Autodesk Inventor part; units mm, degrees
ref_plane "YZ Plane" through (0, 0, 0) normal (1, 0, 0) x (0, 1, 0)
ref_plane "XZ Plane" through (0, 0, 0) normal (0, 1, 0) x (-1, 0, 0)
ref_plane "XY Plane" through (0, 0, 0) normal (0, 0, 1) x (1, 0, 0)
sketch "Sketch1" plane through (0, 0, 0) normal (0, 0, 1) x (1, 0, 0)
  circle A0 centre (15.5, -15.5) radius 2
  circle A1 centre (-15.5, -15.5) radius 2
  circle A2 centre (15.5, 15.5) radius 2
  circle A3 centre (-15.5, 15.5) radius 2
  line L0 (-21.15, 15.4985) -> (-15.4985, 21.15)
  line L1 (-15.4985, 21.15) -> (15.4985, 21.15)
  line L2 (15.4985, 21.15) -> (21.15, 15.4985)
  line L3 (21.15, 15.4985) -> (21.15, -15.4985)
  line L4 (21.15, -15.4985) -> (15.4985, -21.15)
  line L5 (15.4985, -21.15) -> (-15.4985, -21.15)
  line L6 (-15.4985, -21.15) -> (-21.15, -15.4985)
  line L7 (-21.15, -15.4985) -> (-21.15, 15.4985)
  line L8 (28.575, -18.574) -> (28.575, 18.574)
  line L9 (28.575, 18.574) -> (18.574, 28.575)
  line L10 (18.574, 28.575) -> (-18.574, 28.575)
  line L11 (-18.574, 28.575) -> (-28.575, 18.574)
  line L12 (-28.575, 18.574) -> (-28.575, -18.574)
  line L13 (-28.575, -18.574) -> (-18.574, -28.575)
  line L14 (-18.574, -28.575) -> (18.574, -28.575)
  line L15 (18.574, -28.575) -> (28.575, -18.574)
  line L16 (-18.574, -28.575) -> (-145.574, -28.575)
  line L17 (-145.574, -28.575) -> (-145.574, 28.575)
  line L18 (-145.574, 28.575) -> (-18.574, 28.575)
  line L19 (-18.574, 28.575) -> (-18.574, -28.575)
  circle A4 centre (0, 0) radius 11
  dimension "d0" = 127
  dimension "d1" = 57.15
  dimension "d2" = 57.15
extrude "Extrusion1" add sketch "Sketch1" along normal blind 6.35
sketch "Sketch2" plane through (0, 0, 6.35) normal (0, 0, 1) x (1, 0, 0)
  line L0 (-130.4486, -16.3493) -> (-130.4486, -9.9993)
  line L1 (-126.7402, -9.9993) -> (-126.7402, -16.3493)
  line L2 (-130.4486, 9.0507) -> (-130.4486, 15.4007)
  line L3 (-126.7402, 15.4007) -> (-126.7402, 9.0507)
  line L4 (-126.7402, 12.7) -> (-130.4486, 12.7) construction
  line L5 (-126.7402, -12.7) -> (-130.9009, -12.7) construction
  circle A0 centre (-128.5944, 12.7) radius 1.8542
  circle A1 centre (-128.5944, -12.7) radius 1.8542
  dimension "d5" = 3.7084
  dimension "d6" = 3.7084
extrude "Extrusion2" cut sketch "Sketch2" against normal through all
sketch "Sketch3" plane through (0, 0, 6.35) normal (0, 0, 1) x (1, 0, 0)
  line L0 (-145.574, -28.575) -> (-145.574, 28.575)
  line L1 (-151.924, 20.3708) -> (-151.924, 24.0792)
  line L2 (-151.924, -24.5535) -> (-151.924, -20.8451)
  line L3 (-131.1543, 22.225) -> (-145.574, 22.225) construction
  line L4 (-131.1543, -22.225) -> (-145.574, -22.225) construction
  line L5 (-145.574, -20.3708) -> (-132.874, -20.3708)
  line L6 (-132.874, -20.3708) -> (-132.874, -24.0792)
  line L7 (-132.874, -24.0792) -> (-145.574, -24.0792)
  line L8 (-145.574, -24.0792) -> (-145.574, -20.3708)
  line L9 (-145.574, 24.0792) -> (-132.874, 24.0792)
  line L10 (-132.874, 24.0792) -> (-132.874, 20.3708)
  line L11 (-132.874, 20.3708) -> (-145.574, 20.3708)
  line L12 (-145.574, 20.3708) -> (-145.574, 24.0792)
  line L13 (-136.43, 26.162) -> (-139.224, 26.162)
  line L14 (-139.224, 26.162) -> (-139.224, 18.288)
  line L15 (-139.224, 18.288) -> (-136.43, 18.288)
  line L16 (-136.43, 18.288) -> (-136.43, 26.162)
  line L17 (-136.43, -18.288) -> (-139.224, -18.288)
  line L18 (-139.224, -18.288) -> (-139.224, -26.162)
  line L19 (-139.224, -26.162) -> (-136.43, -26.162)
  line L20 (-136.43, -26.162) -> (-136.43, -18.288)
  dimension "d9" = 12.7
  dimension "d10" = 2.794
  dimension "d11" = 7.874
  dimension "d12" = 3.937
  dimension "d13" = 3.937
  dimension "d14" = 7.874
  dimension "d15" = 3.937
  dimension "d16" = 3.937
  dimension "d17" = 6.35
  dimension "d18" = 6.35
  dimension "d19" = 2.794
extrude "Extrusion3" cut sketch "Sketch3" against normal through all
equation "\"d2\" = d1"
equation "\"d12\" = d13"
equation "\"d15\" = d16"
properties part number "tiltColumnNonStepperSide02" material "Titanium"
The model under review builds one solid part; all positions refer to its coordinate system, in mm. A direction names the side the tool comes from. Coordinates: 2 decimals unless noted, no trailing zeros. Write each loop counter-clockwise with the first axis right and the second up, starting at its lowest first coordinate (ties: lowest second). Pieces come first, ordered by that corner, then holes.
1) We need section A-A on x = -15.5. State the section outline as (y, z) points (3 decimals), then the cut area to 3 significant figures.
2) To check wall thickness, follow probe 1 along Y at (x, z) = (15.5, 2.25) (3 decimals); probe 2 along X at (y, z) = (12.7, 4) (3 decimals); probe 3 along X at (y, z) = (15, 4) (1 decimal). State the ranges of each line that lie inside material, in increasing order.
3) We need section B-B on y = 8. State the section outline as (x, z) points (3 decimals), then the cut area to 3 significant figures.
4) We need section C-C on z = 3.75. Count the separate pieces of the cut face and the enclosed holes in it, then the cut area to 3 significant figures.
5) The part is to be moulded in two halves that separate along Y. For faces 4 (the face through (-60, 0, 6.35)), 5 (the face through (-135, -20.371, 3)), 6 (the face through (15.24, 13.517, 3.131)), 7 (the face through (23.504, -23.645, 3.131)), say which applies: pulls with the +Y half, pulls with the -Y half, needs draft (parallel to the pull), parting line crosses it, or undercut.
6) Machinability: for faces 1 (the face through (-138, -18.288, 3)), 2 (the face through (-132.874, -22, 3)), 3 (the face through (28.575, 0, 3)), which of the approach directions +Z, -Z, +X, -X, +Y, -Y give a long, thin tool a straight path to every point of the face, cutting with its end or side? Answer none if there is none.
7) Clearance check with flat-ended pins moving along their axes: pin 1 Ø3 at (y, z) = (22, 3) entering from -X; pin 2 Ø17.5 at (x, y) = (0, 0) entering from +Z; pin 3 Ø0.6 at (y, z) = (-25, 3) entering from +X. State where each tip first meets the part, or that it passes through.
8) We need section D-D on y = -5.5. State the section outline as (x, z) points (3 decimals).
Answer list:
1. outline: (-28.575, 0) - (-17.5, 0) - (-17.5, 6.35) - (-28.575, 6.35) - close; (-13.5, 0) - (13.5, 0) - (13.5, 6.35) - (-13.5, 6.35) - close; (17.5, 0) - (28.575, 0) - (28.575, 6.35) - (17.5, 6.35) - close
1. area: 312 mm2
2. probe 1: y = -28.575 to -17.5, -13.5 to 13.5, 17.5 to 28.575
2. probe 2: x = -145.574 to -130.449, -126.74 to 28.575
2. probe 3: x = -145.6 to -17.4, -13.6 to 13.6, 17.4 to 28.6
3. outline: (-145.574, 0) - (-7.55, 0) - (-7.55, 6.35) - (-145.574, 6.35) - close; (7.55, 0) - (28.575, 0) - (28.575, 6.35) - (7.55, 6.35) - close
3. area: 1,010 mm2
4. separate pieces: 1
4. enclosed holes: 7
4. area: 9,280 mm2
5. face 4: needs draft
5. face 5: undercut
5. face 6: undercut
5. face 7: pulls with the -Y half
6. face 1: +Z, -Z
6. face 2: +Z, -Z, -X
6. face 3: +Z, -Z, +X, +Y, -Y
7. pin 1: stops at x = -132.87
7. pin 2: passes through
7. pin 3: stops at x = 22.45
8. outline: (-145.574, 0) - (-9.526, 0) - (-9.526, 6.35) - (-145.574, 6.35) - close; (9.526, 0) - (28.575, 0) - (28.575, 6.35) - (9.526, 6.35) - close
